Geometry: final body of the model. Coordinates: model frame, mm. Round coordinates to 2 decimals unless told otherwise and drop trailing zeros. Write each loop counter-clockwise with the first axis right and the second up, starting at its lowest first coordinate (ties: lowest second). Pieces come first, ordered by that corner, then holes. Notation, with made-up numbers: M 49,-7 L 107,-7 A24 ccw 107,18 Z; hole C -3,53.25 d2. An arc over 180 degrees is marked long. Answer as CSV lines item,"result". Start each with the question number.
Q1. Ray query, probe 1 along X at (y, z) = (77.5, 2.1); probe 2 along Y at (x, z) = (-30, 0.6); probe 3 along X at (y, z) = (-13.5, 1.55). Return the intervals inside material, ascending.
Q2. Section query B-B on y = 50.8. Output: boundary loops of the cut face in (x, z) (3 decimals).
Q3. Section query D-D on x = -84.5. Output: boundary loops of the cut face in (y, z) (3 decimals), and give its area (3 significant figures).
Q4. Section query A-A on z = 0.7. Give the number of separate pieces and of enclosed holes in the cut face, and give its area (3 significant figures).
Q5. Mould query, pull axis Y, two halves, no side actions, for faces 1 (the flat face through (21, -21, 0)), 2 (the cylindrical face through (73.105, -1.283, 1.565)), 3 (the cylindrical face through (2.658, 48.762, 1.565)), 4 (the cylindrical face through (-22.025, -99.184, 1.565)). Classes: pulls with the +Y half, pulls with the -Y half, needs draft (parallel to the pull), parting line crosses it, or undercut.
Q6. First-contact query: pin 1 (2.5 mm diameter, centred on x = 30.4, y = 0, fed in from -Z); pin 2 (1 mm diameter, centred on x = 48, z = 0.5, fed in from +Y); pin 3 (1 mm diameter, centred on x = -46, z = 1, fed in from +Y). Flat tips, straight axial feed; report the tip coordinate or a pass-through.
```python
from build123d import *

# Parameters (mm, degrees)
SKETCH1_R           = 101.6
BOSS_EXTRUDE1_DEPTH = 3.175
SKETCH2_R           = 25.4
CUT_EXTRUDE1_DEPTH  = 3.175
SKETCH4_R           = 1.5
CUT_EXTRUDE3_DEPTH  = 10
SKETCH5_R           = 3.35
CUT_EXTRUDE4_DEPTH  = 10
SKETCH6_R           = 3.35
CUT_EXTRUDE5_DEPTH  = 10


with BuildPart() as part:
    # Sketch1 → Boss-Extrude1 (new body)
    with BuildSketch(Plane.XY):
        Circle(SKETCH1_R)
    extrude(amount=BOSS_EXTRUDE1_DEPTH)

    # Sketch2 → Cut-Extrude1 (cut)
    with BuildSketch(Plane.XY.offset(3.175)):
        Circle(SKETCH2_R)
    extrude(amount=-CUT_EXTRUDE1_DEPTH, mode=Mode.SUBTRACT)

    # Sketch4 → Cut-Extrude3 (cut)
    with BuildSketch(Plane(origin=(0, 0, 0), x_dir=(-1, 0, 0), z_dir=(0, 0, -1))):
        with Locations((0, 30.399999906)):
            Circle(SKETCH4_R)
        with Locations((30.399999906, 0)):
            Circle(SKETCH4_R)
        with Locations((0, -30.399999906)):
            Circle(SKETCH4_R)
        with Locations((-30.399999906, 0)):
            Circle(SKETCH4_R)
    extrude(amount=-CUT_EXTRUDE3_DEPTH, mode=Mode.SUBTRACT)

    # Sketch5 → Cut-Extrude4 (cut)
    with BuildSketch(Plane(origin=(0, 0, 0), x_dir=(-1, 0, 0), z_dir=(0, 0, -1))):
        with Locations((0, 50.8)):
            Circle(SKETCH5_R)
        with Locations((50.8, 0)):
            Circle(SKETCH5_R)
        with Locations((0, -50.8)):
            Circle(SKETCH5_R)
        with Locations((-50.8, 0)):
            Circle(SKETCH5_R)
    extrude(amount=-CUT_EXTRUDE4_DEPTH, mode=Mode.SUBTRACT)

    # Sketch6 → Cut-Extrude5 (cut)
    with BuildSketch(Plane(origin=(0, 0, 0), x_dir=(-1, 0, 0), z_dir=(0, 0, -1))):
        with Locations((-76.2, 0)):
            Circle(SKETCH6_R)
        with Locations((0, 76.2)):
            Circle(SKETCH6_R)
        with Locations((0, -76.2)):
            Circle(SKETCH6_R)
        with Locations((76.2, 0)):
            Circle(SKETCH6_R)
    extrude(amount=-CUT_EXTRUDE5_DEPTH, mode=Mode.SUBTRACT)


solid = part.part
```
Entries:
1,probe 1,"x = -65.7 to -3.09, 3.09 to 65.7"
1,probe 2,"y = -97.07 to -1.45, 1.45 to 97.07"
1,probe 3,"x = -100.7 to -21.52, 21.52 to 100.7"
2,outline,"M -87.988,0 L -3.35,0 L -3.35,3.175 L -87.988,3.175 Z; M 3.35,0 L 87.988,0 L 87.988,3.175 L 3.35,3.175 Z"
3,outline,"M -56.412,0 L 56.412,0 L 56.412,3.175 L -56.412,3.175 Z"
3,area,"358 mm^2"
4,separate pieces,"1"
4,enclosed holes,"13"
4,area,"30,100 mm^2"
5,face 1,"needs draft"
5,face 2,"undercut"
5,face 3,"undercut"
5,face 4,"parting line crosses it"
6,pin 1,"passes through"
6,pin 2,"stops at y = 89.81"
6,pin 3,"stops at y = 90.84"
